Part model, mm, in its own coordinate system. Face numbers are marked on the shaded views. A direction names the side the tool comes from. Round coordinates to 2 decimals unless told otherwise and drop trailing zeros. Write each loop counter-clockwise with the first axis right and the second up, starting at its lowest first coordinate (ties: lowest second). Pieces come first, ordered by that corner, then holes.
```python
from build123d import *

# Parameters (mm, degrees)
SKETCH1_W           = 25
SKETCH1_H           = 24
BOSS_EXTRUDE1_DEPTH = 1
SKETCH2_R           = 1.15
CUT_EXTRUDE1_DEPTH  = 1
SKETCH3_W           = 8
SKETCH3_H           = 5
BOSS_EXTRUDE2_DEPTH = 2
SKETCH4_W           = 8
SKETCH4_H           = 8
BOSS_EXTRUDE3_DEPTH = 3
SKETCH5_R           = 3.75
BOSS_EXTRUDE4_DEPTH = 1
SKETCH6_R           = 2.75
BOSS_EXTRUDE5_DEPTH = 1
SKETCH7_R           = 0.75
CUT_EXTRUDE3_DEPTH  = 1
CHAMFER1_SIZE       = 0.5
FILLET2_R           = 0.7
BOSS_EXTRUDE6_DEPTH = 2
SKETCH9_W           = 24
SKETCH9_H           = 1
BOSS_EXTRUDE7_DEPTH = 0.1


with BuildPart() as part:
    # Sketch1 → Boss-Extrude1 (new body)
    with BuildSketch(Plane(origin=(0, 0, 0), x_dir=(1, 0, 0), z_dir=(0, 1, 0))):
        Rectangle(SKETCH1_W, SKETCH1_H)
    extrude(amount=BOSS_EXTRUDE1_DEPTH)

    # Sketch2 → Cut-Extrude1 (cut)
    with BuildSketch(Plane(origin=(0, 1, 0), x_dir=(1, 0, 0), z_dir=(0, 1, 0))):
        with Locations(Location((10.5, -10, 0), (0, 0, 270))):
            Circle(SKETCH2_R)
        with Locations(Location((-10.5, -10, 0), (0, 0, 270))):
            Circle(SKETCH2_R)
        with Locations(Location((-10.5, 2.5, 0), (0, 0, 270))):
            Circle(SKETCH2_R)
        with Locations(Location((10.5, 2.5, 0), (0, 0, 270))):
            Circle(SKETCH2_R)
    extrude(amount=-CUT_EXTRUDE1_DEPTH, mode=Mode.SUBTRACT)

    # Sketch3 → Boss-Extrude2 (add)
    with BuildSketch(Plane(origin=(0, 1, 0), x_dir=(1, 0, 0), z_dir=(0, 1, 0))):
        with Locations((0, -8.293334271)):
            Rectangle(SKETCH3_W, SKETCH3_H)
    extrude(amount=BOSS_EXTRUDE2_DEPTH)

    # Sketch4 → Boss-Extrude3 (add)
    with BuildSketch(Plane(origin=(0, 1, 0), x_dir=(1, 0, 0), z_dir=(0, 1, 0))):
        with Locations((0, 2.5)):
            Rectangle(SKETCH4_W, SKETCH4_H)
    extrude(amount=BOSS_EXTRUDE3_DEPTH)

    # Sketch5 → Boss-Extrude4 (add)
    with BuildSketch(Plane(origin=(0, 4, 0), x_dir=(1, 0, 0), z_dir=(0, 1, 0))):
        with Locations(Location((0, 2.5, 0), (0, 0, 270))):
            Circle(SKETCH5_R)
    extrude(amount=BOSS_EXTRUDE4_DEPTH)

    # Sketch6 → Boss-Extrude5 (add)
    with BuildSketch(Plane(origin=(0, 5, 0), x_dir=(1, 0, 0), z_dir=(0, 1, 0))):
        with Locations(Location((0, 2.5, 0), (0, 0, 270))):
            Circle(SKETCH6_R)
    extrude(amount=BOSS_EXTRUDE5_DEPTH)

    # Sketch7 → Cut-Extrude3 (cut)
    with BuildSketch(Plane(origin=(0, 6, 0), x_dir=(1, 0, 0), z_dir=(0, 1, 0))):
        with Locations(Location((0, 2.5, 0), (0, 0, 270))):
            Circle(SKETCH7_R)
    extrude(amount=-CUT_EXTRUDE3_DEPTH, mode=Mode.SUBTRACT)

    # Chamfer1
    chamfer1_edges = [part.edges().sort_by_distance(p)[0] for p in [
        (0, 6, -3.25),
    ]]
    chamfer(chamfer1_edges, length=CHAMFER1_SIZE)

    # Fillet2
    # the kernel refuses this fillet: 0.7 mm, written as the material it adds along each edge
    with BuildSketch(Plane(origin=(0, 5, -2.5), x_dir=(0, 0, 1), z_dir=(-1, 0, 0))) as fillet2_piece_1:
        with BuildLine():
            CenterArc((0.079179607, 0.7), FILLET2_R, 270, 73.398450401)
            Line((0.079179607, 0), (0.079179607, -0.014))
            Line((0.079179607, -0.014), (0.75, -0.014))
            Line((0.75, -0.014), (0.764, 0))
            ThreePointArc((0.764, 0), (0.764, 0.25), (0.763416408, 0.496))
            Line((0.763416408, 0.496), (0.75, 0.5))
        make_face()
    revolve(axis=Axis((0, 5, -2.5), (0, 1, 0)))

    # Sketch8 → Boss-Extrude6 (add)
    with BuildSketch(Plane.XZ):
        Polygon((10.5, -11.875), (12, -11.875), (12, -10.875), (10.5, -10.875), (10.5, -6.625), (-10.5, -6.625), (-10.5, -10.875), (-12, -10.875), (-12, -11.875), (-10.5, -11.875), align=None)
    extrude(amount=BOSS_EXTRUDE6_DEPTH)

    # Sketch9 → Boss-Extrude7 (add)
    with BuildSketch(Plane.XZ.offset(2)):
        with Locations((0, -11.375)):
            Rectangle(SKETCH9_W, SKETCH9_H)
    extrude(amount=BOSS_EXTRUDE7_DEPTH)


solid = part.part
```
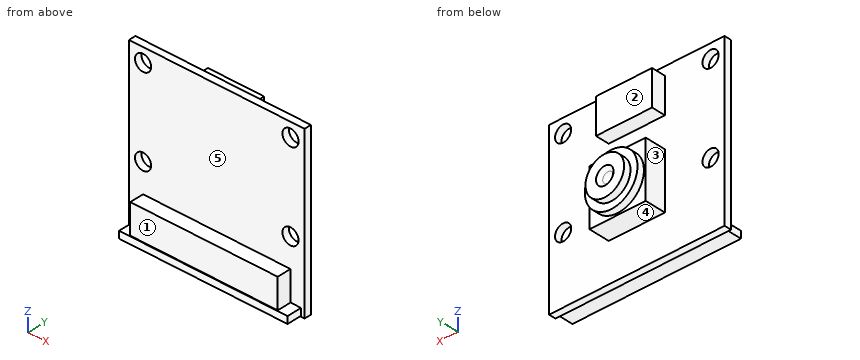
Q1. Cut at A-A on z = 10. Write the cut outline in (x, y).
Values follow:
outline: (-12.5, 0) - (-11.65, 0) - (-11.65, 1) - (-12.5, 1) - close; (-9.35, 0) - (9.35, 0) - (9.35, 1) - (4, 1) - (4, 3) - (-4, 3) - (-4, 1) - (-9.35, 1) - close; (11.65, 0) - (12.5, 0) - (12.5, 1) - (11.65, 1) - close
Q2. Mould opens along Z. For the marked faces 4 and 5 say: +Z half, -Z half, draft (parallel to the pull), parting line (faces both ways), or undercut.
Values follow:
face 4: -Z half
face 5: draft
Q3. Drop flat-ended pins along their axis: pin 1 (1.5 mm diameter, centred on y = 2.5, z = 9, fed in from -X); pin 2 (0.9 mm diameter, centred on x = 1, y = 3, fed in from +Z); pin 3 (3.5 mm diameter, centred on x = 10.5, z = -2.5, fed in from +Y); pin 4 (9 mm diameter, centred on x = -0.5, z = -2.5, fed in from +Y). Give the stop position or say it passes through.
Values follow:
pin 1: stops at x = -4
pin 2: stops at z = 10.79
pin 3: stops at y = 1
pin 4: stops at y = 6
Q4. Cut at D-D on x = -8. Write the cut outline in (y, z) (3 decimals), plus the area to 3 significant figures.
Values follow:
outline: (-2.1, -11.875) - (0, -11.875) - (0, -12) - (1, -12) - (1, 12) - (0, 12) - (0, -6.625) - (-2, -6.625) - (-2, -10.875) - (-2.1, -10.875) - close
area: 34.6 mm2
Q5. Which spindle directions (+Z, -Z, +X, -X, +Y, -Y) get a long thin tool onto all of the face, cutting with end or side? Do the marked faces 1, 2 and 3. Say none if no direction does.
Values follow:
face 1: +Z, +X, -X, -Y
face 2: +Z, +X, -X, +Y
face 3: +Z, -Z, -X, +Y
Q6. Wall check: L1, parallel to X at y = 0.25, z = -2.5; L2, parallel to Z at x = 0.75, y = 2.25; L3, parallel to Y at x = -2, z = -10.5. Give the ranges that are in metal, low to high.
Values follow:
L1: x = -12.5 to -11.65, -9.35 to 9.35, 11.65 to 12.5
L2: z = -6.5 to 1.5, 5.79 to 10.79
L3: y = -2 to 1
Q7. Cut at C-C on y = 0.5. Write the cut outline in (x, z).
Values follow:
outline: (-12.5, -12) - (12.5, -12) - (12.5, 12) - (-12.5, 12) - close; hole circle Ø2.3 at (-10.5, -2.5); hole circle Ø2.3 at (-10.5, 10); hole circle Ø2.3 at (10.5, -2.5); hole circle Ø2.3 at (10.5, 10)
Q8. Cut at B-B on y = 2.25. Write the cut outline in (x, z).
Values follow:
outline: (-4, -6.5) - (4, -6.5) - (4, 1.5) - (-4, 1.5) - close; (-4, 5.79) - (4, 5.79) - (4, 10.79) - (-4, 10.79) - close
